```python
from build123d import *

# Parameters (mm, degrees)
SCHIZZO1_W                           = 25
SCHIZZO1_H                           = 25
ESTRUSIONE_ESTRUSIONE1_DEPTH         = 8
SCHIZZO8_R                           = 5
ESTRUSIONE_ESTRUSIONE3_DEPTH         = 15
RACCORDO1_R                          = 3
TAGLIO_ESTRUSIONE2_REACH             = 25
SCHIZZO9_R                           = 1.6
SCHIZZO10_R                          = 3
TAGLIO_ESTRUSIONE3_DEPTH             = 4
SCHIZZO11_R                          = 3
TAGLIO_ESTRUSIONE4_DEPTH             = 16
TAGLIO_ESTRUSIONE6_REACH             = 25
SCHIZZO13_R                          = 1.6
TAGLIO_ESTRUSIONE8_START             = -3
TAGLIO_ESTRUSIONE8_DEPTH             = 19
RIPETIZIONECIRCOLARE1_COUNT          = 2
RIPETIZIONECIRCOLARE1_ANGLE          = 180
TAGLIO_ESTRUSIONE9_REACH             = 10
TAGLIO_ESTRUSIONE9_DIRECTION_2_REACH = 17
RACCORDO2_R                          = 3
RACCORDO3_R                          = 3
RACCORDO4_R                          = 8


with BuildPart() as part:
    # Schizzo1 → Estrusione-Estrusione1 (new body)
    with BuildSketch(Plane.XY):
        Rectangle(SCHIZZO1_W, SCHIZZO1_H)
    extrude(amount=ESTRUSIONE_ESTRUSIONE1_DEPTH)

    # Schizzo8 → Estrusione-Estrusione3 (add)
    with BuildSketch(Plane.XY.offset(8)):
        Circle(SCHIZZO8_R)
    extrude(amount=ESTRUSIONE_ESTRUSIONE3_DEPTH)

    # Raccordo1
    raccordo1_edges = [part.edges().sort_by_distance(p)[0] for p in [
        (-5, 0, 8),
    ]]
    fillet(raccordo1_edges, radius=RACCORDO1_R)

    # Schizzo9 → Taglio-Estrusione2 (cut, up to next)
    with BuildSketch(Plane(origin=(0, 0, 0), x_dir=(-1, 0, 0), z_dir=(0, 0, -1)), mode=Mode.PRIVATE) as taglio_estrusione2_sk1:
        Circle(SCHIZZO9_R)
    taglio_estrusione2_tool1 = extrude(taglio_estrusione2_sk1.sketch, amount=-TAGLIO_ESTRUSIONE2_REACH, mode=Mode.PRIVATE) & part.part
    add(taglio_estrusione2_tool1.solids().sort_by_distance((0, 0, 0))[0], mode=Mode.SUBTRACT)

    # Schizzo10 → Taglio-Estrusione3 (cut)
    with BuildSketch(Plane(origin=(0, 0, 0), x_dir=(-1, 0, 0), z_dir=(0, 0, -1))):
        Circle(SCHIZZO10_R)
    extrude(amount=-TAGLIO_ESTRUSIONE3_DEPTH, mode=Mode.SUBTRACT)

    # Schizzo11 → Taglio-Estrusione4 (cut)
    with BuildSketch(Plane.XY.offset(23)):
        Circle(SCHIZZO11_R)
    extrude(amount=-TAGLIO_ESTRUSIONE4_DEPTH, mode=Mode.SUBTRACT)

    # Schizzo13 → Taglio-Estrusione6 (cut, up to next)
    with BuildSketch(Plane(origin=(0, 0, 0), x_dir=(-1, 0, 0), z_dir=(0, 0, -1)), mode=Mode.PRIVATE) as taglio_estrusione6_sk1:
        with Locations((-8.485281374, -8.485281374)):
            Circle(SCHIZZO13_R)
    taglio_estrusione6_tool1 = extrude(taglio_estrusione6_sk1.sketch, amount=-TAGLIO_ESTRUSIONE6_REACH, mode=Mode.PRIVATE) & part.part
    add(taglio_estrusione6_tool1.solids().sort_by_distance((8.485281, -8.485281, 0))[0], mode=Mode.SUBTRACT)
    # Schizzo13 → Taglio-Estrusione6 (cut, up to next)
    with BuildSketch(Plane(origin=(0, 0, 0), x_dir=(-1, 0, 0), z_dir=(0, 0, -1)), mode=Mode.PRIVATE) as taglio_estrusione6_sk2:
        with Locations((8.485281374, 8.485281374)):
            Circle(SCHIZZO13_R)
    taglio_estrusione6_tool2 = extrude(taglio_estrusione6_sk2.sketch, amount=-TAGLIO_ESTRUSIONE6_REACH, mode=Mode.PRIVATE) & part.part
    add(taglio_estrusione6_tool2.solids().sort_by_distance((-8.485281, 8.485281, 0))[0], mode=Mode.SUBTRACT)

    # Schizzo17 → Taglio-Estrusione8 (cut)
    with BuildSketch(Plane.XY.offset(8).offset(TAGLIO_ESTRUSIONE8_START)):
        with BuildLine():
            Line((4.5, -12.5), (4.5, -8.5))
            ThreePointArc((4.5, -8.5), (5.671572875, -5.671572875), (8.5, -4.5))
            Line((8.5, -4.5), (12.5, -4.5))
            Line((12.5, -4.5), (12.5, -12.5))
            Line((12.5, -12.5), (4.5, -12.5))
        make_face()
    taglio_estrusione8 = extrude(amount=TAGLIO_ESTRUSIONE8_DEPTH, mode=Mode.SUBTRACT)

    # RipetizioneCircolare1: Taglio-Estrusione8 ×2 about axis
    ripetizionecircolare1_axis = Axis((0, 0, 0), (0, 0, 1))
    for i in range(1, RIPETIZIONECIRCOLARE1_COUNT):
        add(taglio_estrusione8.rotate(ripetizionecircolare1_axis, i * RIPETIZIONECIRCOLARE1_ANGLE / (RIPETIZIONECIRCOLARE1_COUNT - 1)), mode=Mode.SUBTRACT)

    # Schizzo20 → Taglio-Estrusione9 (cut, up to next)
    with BuildSketch(Plane.XY.offset(8), mode=Mode.PRIVATE) as taglio_estrusione9_sk1:
        with BuildLine():
            Line((-12.5, -12.5), (4.5, -12.5))
            ThreePointArc((4.5, -12.5), (0.853575925, -12.104324481), (-2.623106886, -10.935716643))
            ThreePointArc((-2.623106886, -10.935716643), (-5.428932188, -5.428932188), (-10.935716643, -2.623106886))
            ThreePointArc((-10.935716643, -2.623106886), (-12.104324481, 0.853575925), (-12.5, 4.5))
            Line((-12.5, 4.5), (-12.5, -12.5))
        make_face()
    taglio_estrusione9_tool1 = extrude(taglio_estrusione9_sk1.sketch, amount=-TAGLIO_ESTRUSIONE9_REACH, mode=Mode.PRIVATE) & part.part
    add(taglio_estrusione9_tool1.solids().sort_by_distance((-8.104879, -8.104879, 8))[0], mode=Mode.SUBTRACT)

    # Schizzo20 → Taglio-Estrusione9 direction 2 (cut, up to next)
    with BuildSketch(Plane.XY.offset(8), mode=Mode.PRIVATE) as taglio_estrusione9_direction_2_sk1:
        with BuildLine():
            Line((-12.5, -12.5), (4.5, -12.5))
            ThreePointArc((4.5, -12.5), (0.853575925, -12.104324481), (-2.623106886, -10.935716643))
            ThreePointArc((-2.623106886, -10.935716643), (-5.428932188, -5.428932188), (-10.935716643, -2.623106886))
            ThreePointArc((-10.935716643, -2.623106886), (-12.104324481, 0.853575925), (-12.5, 4.5))
            Line((-12.5, 4.5), (-12.5, -12.5))
        make_face()
    taglio_estrusione9_direction_2_tool1 = extrude(taglio_estrusione9_direction_2_sk1.sketch, amount=TAGLIO_ESTRUSIONE9_DIRECTION_2_REACH, mode=Mode.PRIVATE) & part.part
    add(taglio_estrusione9_direction_2_tool1.solids().sort_by_distance((-8.104879, -8.104879, 8))[0], mode=Mode.SUBTRACT)

    # Raccordo2
    raccordo2_edges = [part.edges().sort_by_distance(p)[0] for p in [
        (-10.935716643, -2.623106886, 4),
        (-2.623106886, -10.935716643, 4),
    ]]
    fillet(raccordo2_edges, radius=RACCORDO2_R)

    # Raccordo3
    raccordo3_edges = [part.edges().sort_by_distance(p)[0] for p in [
        (12.5, -12.5, 2.5),
        (-12.5, 12.5, 2.5),
    ]]
    fillet(raccordo3_edges, radius=RACCORDO3_R)

    # Raccordo4
    raccordo4_edges = [part.edges().sort_by_distance(p)[0] for p in [
        (12.5, 12.5, 4),
    ]]
    fillet(raccordo4_edges, radius=RACCORDO4_R)


solid = part.part
```
Geometry: final body of the model. Coordinates: model frame, mm. A direction names the side the tool comes from. Give positions to 0.01 mm unless a question says otherwise; leave off trailing zeros. Order: outer loops, then holes, each group sorted by start corner. A loop starts at its lowest first (then second) coordinate and runs counter-clockwise, first axis right, second up. Notation, with made-up numbers: (73.5, 53) -> (88.5, 53) arc R16 cw to (88.5, 76) -> close; hole circle Ø7 at (34.5, 48.25). An arc over 180 degrees is marked (long way). Write each question's results on one line, items separated by ' | '. Start each with the question number.
1) Draft query along X for faces 5 (the flat face through (-10.3, 8.4, 5)), 6 (the flat face through (-1.3, -1.3, 4)), 7 (the cylindrical face through (-11.6, 11.64, 2.54)). Return one class per face: pulls with the +X half, pulls with the -X half, needs draft (parallel to the pull), parting line crosses it, or undercut.
2) Section C-C (z = 17.25). Return loops of the section in (x, y), then the cut area to 3 significant figures.
3) First-contact query: pin 1 (3.5 mm diameter, centred on x = 10, z = 7, fed in from -Y); pin 2 (3.5 mm diameter, centred on y = -10.5, z = 6.5, fed in from +X); pin 3 (4 mm diameter, centred on x = -7.5, y = 10.5, fed in from +Z). Flat tips, straight axial feed; report the tip coordinate or a pass-through.
4) Set-up query: faces 1 (the flat face through (-10, 4.5, 6)), 2 (the cylindrical face through (3, 0, 2)), 3 (the flat face through (4.5, -11, 6)), 4 (the flat face through (1.3, -1.3, 7)). Return all of +Z, -Z, +X, -X, +Y, -Y with unobstructed straight access to the full face (end or side cutting, diameter ignored); none if empty.
5) Line query: line 1 (Y direction, x = 0, z = 18); line 2 (X direction, y = 0.75, z = 9.25); line 3 (Z direction, x = -2, y = 0.75). Output: solid intervals per line, ascending. Write a range as from..to.
6) Section D-D (z = 3.25). Count the separate pieces of the cut face and the enclosed holes in it, then the cut area to 3 significant figures.
7) Section A-A (y = 0). Return loops of the section in (x, z), then the cut area to 3 significant figures.
Calculated:
1) face 5: needs draft | face 6: undercut | face 7: pulls with the -X half
2) outline: circle Ø10 at (0, 0); hole circle Ø6 at (0, 0) | area: 50.3 mm2
3) pin 1: y = -4.51 | pin 2: x = 12.5 | pin 3: z = 5
4) face 1: +Z, -X, +Y | face 2: -Z | face 3: +Z, +X, -Y | face 4: +Z
5) line 1: -5..-3, 3..5 | line 2: -5.51..-2.9, 2.9..5.51 | line 3: 4..7
6) separate pieces: 1 | enclosed holes: 3 | area: 477 mm2
7) outline: (-11.89, 0) -> (-3, 0) -> (-3, 4) -> (-1.6, 4) -> (-1.6, 7) -> (-3, 7) -> (-3, 23) -> (-5, 23) -> (-5, 11) arc R3 cw to (-8, 8) -> (-11.89, 8) -> close; (1.6, 4) -> (3, 4) -> (3, 0) -> (12.5, 0) -> (12.5, 8) -> (8, 8) arc R3 cw to (5, 11) -> (5, 23) -> (3, 23) -> (3, 7) -> (1.6, 7) -> close | area: 219 mm2
